Could you check a few things on this model? Use its own coordinates, in mm. Face numbers are marked on the shaded views. A direction names the side the tool comes from. Round coordinates to 2 decimals unless told otherwise and drop trailing zeros. Write each loop counter-clockwise with the first axis right and the second up, starting at its lowest first coordinate (ties: lowest second). Pieces come first, ordered by that corner, then holes. Notation, with made-up numbers: (-1, 72) - (16, 72) arc R28 cw to (16, 90) - close; hole circle Ø1 at (31.5, 44.5). An arc over 180 degrees is marked (long way). Put each result on its own line as item: value.
from build123d import *

# Parameters (mm, degrees)
SKETCH2_W           = 20
SKETCH2_H           = 10
BOSS_EXTRUDE1_DEPTH = 9


with BuildPart() as part:
    # Sketch1 → Revolve1 (revolve)
    with BuildSketch(Plane.XY):
        Polygon((11.05, 0), (2.375, 0), (2.375, -0.2), (3.05, -0.2), (3.05, -2.378460969), (1.85, -2.7), (1.85, -6.3), (1.15, -7), (0, -7), (0, -9), (11.05, -9), align=None)
    revolve(axis=Axis((0, 0, 0), (0, 1, 0)))

    # Sketch2 → Boss-Extrude1 (add)
    with BuildSketch(Plane(origin=(0, 0, 0), x_dir=(1, 0, 0), z_dir=(0, 1, 0))):
        with Locations((0, -9.701329599)):
            Rectangle(SKETCH2_W, SKETCH2_H)
    extrude(amount=-BOSS_EXTRUDE1_DEPTH)


solid = part.part
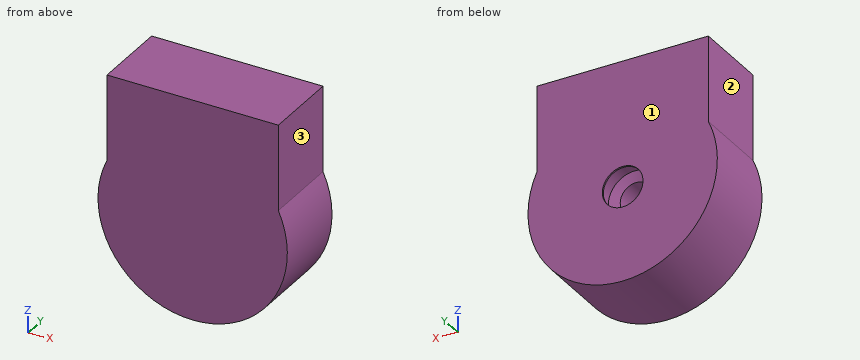
(1) Imagine slicing it at B-B, the plane z = 0. List the corners of the cut face in (x, y) for me (3 decimals).
Values found:
outline: (-11.05, -9) - (11.05, -9) - (11.05, 0) - (2.375, 0) - (2.375, -0.2) - (3.05, -0.2) - (3.05, -2.378) - (1.85, -2.7) - (1.85, -6.3) - (1.15, -7) - (-1.15, -7) - (-1.85, -6.3) - (-1.85, -2.7) - (-3.05, -2.378) - (-3.05, -0.2) - (-2.375, -0.2) - (-2.375, 0) - (-11.05, 0) - close
(2) Please list where these lines run through material, in increasing order: probe 1 along Z at (x, y) = (0, -0.1) (3 decimals); probe 2 along X at (y, z) = (-5.05, 0); probe 3 along X at (y, z) = (-0.05, 0) (3 decimals). Write a range as from..to.
Values found:
probe 1: z = -11.05..-2.375, 2.375..14.701
probe 2: x = -11.05..-1.85, 1.85..11.05
probe 3: x = -11.05..-2.375, 2.375..11.05
(3) Imagine slicing it at C-C, the plane y = -1.75. List the corners of the cut face in (x, z) for me, then the cut area to 3 significant figures.
Values found:
outline: (-10, 4.7) arc R11.05 ccw (long way) to (10, 4.7) - (10, 14.7) - (-10, 14.7) - close; hole circle Ø6.1 at (0, 0)
area: 463 mm^2
(4) I'm going to push flat-ended pins straight in: pin 1 (0.7 mm diameter, centred on x = 0.5, z = 0, fed in from +Y); pin 2 (4 mm diameter, centred on x = -8.5, y = -3, fed in from -Z); pin 3 (3 mm diameter, centred on x = 0, z = 0, fed in from +Y). Where does each tip first touch, or does it pass through?
Values found:
pin 1: stops at y = -7
pin 2: stops at z = -8.94
pin 3: stops at y = -6.65
(5) Imagine slicing it at D-D, the plane x = 9. List the corners of the cut face in (y, z) for me.
Values found:
outline: (-9, -6.41) - (0, -6.41) - (0, 14.7) - (-9, 14.7) - close
(6) For the marked faces 1, 2 and 3, which set-ups out of +Z, -Z, +X, -X, +Y, -Y let a thin tool reach every point of the face, with its end or its side?
Values found:
face 1: +Z, -Z, +X, -X, +Y
face 2: +Z, -X, +Y, -Y
face 3: +Z, +X, +Y, -Y
(7) Imagine slicing it at A-A, the plane y = -3.5. List the corners of the cut face in (x, z) for me, then the cut area to 3 significant figures.
Values found:
outline: (-10, 4.7) arc R11.05 ccw (long way) to (10, 4.7) - (10, 14.7) - (-10, 14.7) - close; hole circle Ø3.7 at (0, 0)
area: 482 mm^2
